The listing builds one solid part. Answer for the finished solid, in the listing's coordinates (mm). A direction names the side the tool comes from. Round coordinates to 2 decimals unless told otherwise and drop trailing zeros. Order: outer loops, then holes, each group sorted by start corner. A loop starts at its lowest first (then second) coordinate and runs counter-clockwise, first axis right, second up. Notation, with made-up numbers: (-24, 4.25) - (9, 4.25) arc R15 ccw to (9, 9.25) - close; hole circle Ø11 at (-26.5, 60). An arc over 180 degrees is marked (long way). One line per item, written item: value. Start each with the question number.
1. Straight lines are drawn through the part: line 1 (Y direction, x = 45.25, z = 0); line 2 (X direction, y = -3.5, z = 0); line 3 (Z direction, x = 49, y = -1.5). For each, find the intervals that lie inside material, in ascending order.
2. Section B-B, the plane x = 49 is taken. Give the vertices of the cut face in (y, z), then the cut area to 3 significant figures.
3. Section A-A, the plane x = 43 is taken. Give the vertices of the cut face in (y, z).
4. For a pull along Y with two mould halves and no side action, classify faces 3 (the flat face through (55, 0, 0)), 4 (the flat face through (57.25, 2.13, -3.77)), 5 (the flat face through (57.25, -2.13, 3.77)), 6 (the cylindrical face through (44.29, -3.13, -0.54)) as released by +Y, released by -Y, zero draft, split by the parting line, or undercut.
5. Flat-ended cylindrical pins translate along their axes: P1, Ø2.5, axis at x = 43, z = 0, coming from the -Y side; P2, Ø3, axis at y = 0, z = 0, coming from the -X side. Find the tip coordinate at first contact, or state that the pin passes through.
6. Section D-D, the plane y = 0.5 is taken. Give the vertices of the cut face in (x, z) (3 decimals).
7. Section C-C, the plane z = 0 is taken. Give the vertices of the cut face in (x, y), then the cut area to 3 significant figures.
8. A tool of negligible diameter and unlimited length cuts with its end or side. For faces 1 (the flat face through (57.25, 2.2, 3.73)), 2 (the cylindrical face through (52.535, -0.024, 1.405)), from which of +Z, -Z, +X, -X, +Y, -Y can it reach the whole face along a straight path? Write none if from no direction.
from build123d import *

# Parameters (mm, degrees)
SKETCH205_R          = 1.4
PAD127041_DEPTH      = 10
SKETCH175_R          = 2.35
PAD127013_DEPTH      = 100
PAD127012_DEPTH      = 100
PAD127040_DEPTH      = 20
PAD127040_DEPTH_BACK = 16


with BuildPart() as setscrewcutout:
    # Sketch205 → Pad127041 (new body, symmetric)
    with BuildSketch(Plane(origin=(55, 0, 0), x_dir=(1, 0, 0), z_dir=(0, -1, 0))):
        with Locations((-12, 0)):
            Circle(SKETCH205_R)
    extrude(amount=PAD127041_DEPTH, both=True)


with BuildPart() as obj1:
    # Sketch175 → Pad127013 (new body)
    with BuildSketch(Plane.YZ.offset(50)):
        Circle(SKETCH175_R)
    extrude(amount=-PAD127013_DEPTH)


with BuildPart() as axlecutout:
    # Sketch176 → Pad127012 (new body)
    with BuildSketch(Plane.YZ.offset(55)):
        with BuildLine():
            ThreePointArc((-1.74356, 1.5), (0, -2.3), (1.74356, 1.5))
            ThreePointArc((-1.74356, 1.5), (0, 1.404716), (1.74356, 1.5))
        make_face()
    extrude(amount=-PAD127012_DEPTH)

    # Fusion004020013: union obj1
    add(obj1.part)


with BuildPart() as adapteraxle:
    # Sketch204 → Pad127040 (new body, two sides)
    with BuildSketch(Plane.YZ.offset(55)) as pad127040_sk:
        Polygon((4.330127, 2.5), (0, 5), (-4.330127, 2.5), (-4.330127, -2.5), (0, -5), (4.330127, -2.5), align=None)
    extrude(amount=PAD127040_DEPTH)
    extrude(pad127040_sk.sketch, amount=-PAD127040_DEPTH_BACK)

    # Cut007019024: cut AxleCutout
    add(axlecutout.part, mode=Mode.SUBTRACT)

    # Cut007019025: cut SetScrewCutout
    add(setscrewcutout.part, mode=Mode.SUBTRACT)


solid = adapteraxle.part
Answer list:
1. line 1: y = -4.33 to -2.35, 2.35 to 4.33
1. line 2: x = 39 to 41.6, 44.4 to 75
1. line 3: z = -4.13 to -1.81, 1.81 to 4.13
2. outline: (-4.33, -2.5) - (0, -5) - (4.33, -2.5) - (4.33, 2.5) - (0, 5) - (-4.33, 2.5) - close; hole circle Ø4.7 at (0, 0)
2. area: 47.6 mm²
3. outline: (-4.33, -2.5) - (0, -5) - (4.33, -2.5) - (4.33, -1.4) - (1.89, -1.4) arc R2.35 cw to (-1.89, -1.4) - (-4.33, -1.4) - close; (-4.33, 1.4) - (-1.89, 1.4) arc R2.35 cw to (1.89, 1.4) - (4.33, 1.4) - (4.33, 2.5) - (0, 5) - (-4.33, 2.5) - close
4. face 3: undercut
4. face 4: released by +Y
4. face 5: released by -Y
4. face 6: zero draft
5. P1: passes through
5. P2: stops at x = 50
6. outline: (39, -4.711) - (75, -4.711) - (75, 4.711) - (39, 4.711) - (39, 2.296) - (50, 2.296) - (50, 1.413) - (55, 1.413) - (55, -2.245) - (50, -2.245) - (50, -2.296) - (39, -2.296) - close
7. outline: (39, -4.33) - (41.6, -4.33) - (41.6, -2.35) - (39, -2.35) - close; (39, 2.35) - (41.6, 2.35) - (41.6, 4.33) - (39, 4.33) - close; (44.4, -4.33) - (75, -4.33) - (75, 4.33) - (44.4, 4.33) - (44.4, 2.35) - (50, 2.35) - (50, 2.3) - (55, 2.3) - (55, -2.3) - (50, -2.3) - (50, -2.35) - (44.4, -2.35) - close
7. area: 226 mm²
8. face 1: +Z, +X, -X, +Y
8. face 2: -X
